Study the drawing (mm; zero at the part's minimum x, y, z) and answer. A direction names the side the tool comes from. Give positions to 0.01 mm unless a question says otherwise; leave off trailing zeros. Order: outer loops, then holes, each group sorted by start corner. A loop starts at its lowest first (then second) coordinate and runs counter-clockwise, first axis right, second up.
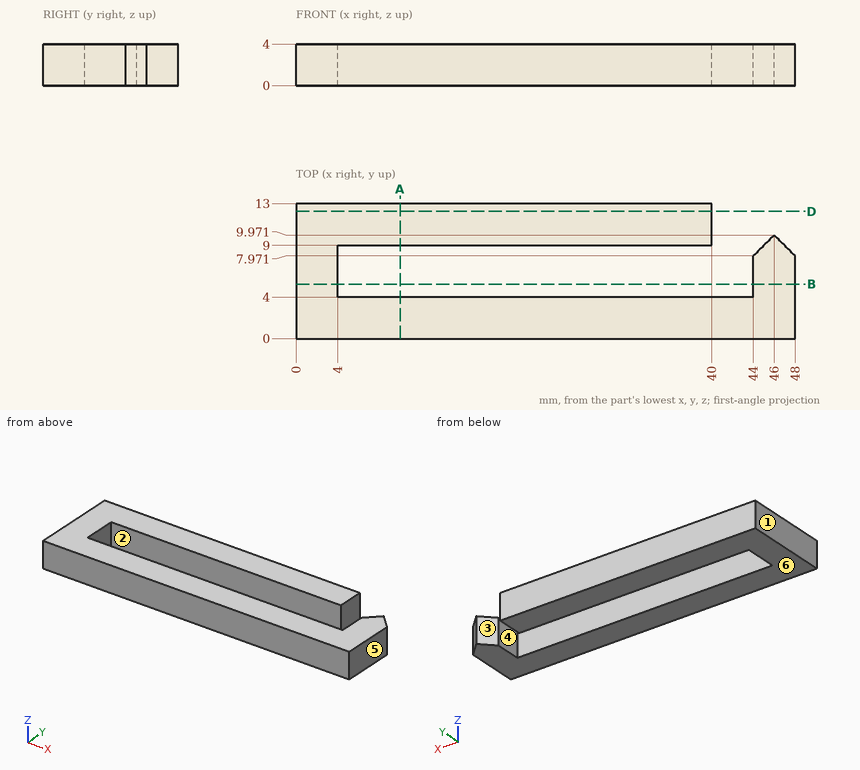
1) Straight lines are drawn through the part: probe 1 along X at (y, z) = (6.5, 1.2); probe 2 along Y at (x, z) = (30, 2); probe 3 along X at (y, z) = (11.25, 0.7). For each, find the intervals that lie inside material, in ascending order.
Geometry says:
probe 1: x = 0 to 4, 44 to 48
probe 2: y = 0 to 4, 9 to 13
probe 3: x = 0 to 40
2) A tool of negligible diameter and unlimited length cuts with its end or side. For the marked faces 1, 2 and 3, from which of +Z, -Z, +X, -X, +Y, -Y can it reach the whole face along a straight path? Write none if from no direction.
Geometry says:
face 1: +Z, -Z, -X, +Y, -Y
face 2: +Z, -Z
face 3: +Z, -Z, +Y
3) Find section B-B (y = 5.25). Write down the section's boundary in (x, z).
Geometry says:
outline: (0, 0) - (4, 0) - (4, 4) - (0, 4) - close; (44, 0) - (48, 0) - (48, 4) - (44, 4) - close
4) For a pull along X with two mould halves and no side action, classify the marked faces 4, 5 and 6 as +X half, -X half, draft (parallel to the pull), parting line (faces both ways), or undercut.
Geometry says:
face 4: undercut
face 5: +X half
face 6: draft
5) Given P1, Ø1.2, axis at y = 10.5, z = 3, coming from the +X side, flat-ended and moving along its own axis, determine where the tip first touches the part or whether it passes through.
Geometry says:
P1: stops at x = 46.07
6) Find section D-D (y = 12.25). Write down the section's boundary in (x, z), then the cut area to 3 significant figures.
Geometry says:
outline: (0, 0) - (40, 0) - (40, 4) - (0, 4) - close
area: 160 mm2
7) Find section A-A (x = 10). Write down the section's boundary in (y, z).
Geometry says:
outline: (0, 0) - (4, 0) - (4, 4) - (0, 4) - close; (9, 0) - (13, 0) - (13, 4) - (9, 4) - close
